```python
from build123d import *

# Parameters (mm, degrees)
SKETCH_1_W          = 12
SKETCH_1_H          = 10
EXTRUDE_1_DEPTH     = 9
FILLET_1_R          = 0.5
SKETCH_2_R          = 2
SKETCH_2_R_2        = 1.5
EXTRUDE_2_DEPTH     = 0.8
FILLET_2_R          = 0.05
SKETCH_7_R          = 2
CUT_EXTRUDE_4_DEPTH = 0.1


with BuildPart() as part:
    # 草图1 → 凸台-拉伸1 (new body)
    with BuildSketch(Plane.XY):
        Rectangle(SKETCH_1_W, SKETCH_1_H)
    extrude(amount=EXTRUDE_1_DEPTH)

    # 圆角1
    fillet_1_edges = [part.edges().sort_by_distance(p)[0] for p in [
        (6, -5, 4.5),
        (-6, -5, 4.5),
        (-6, 5, 4.5),
        (6, 5, 4.5),
    ]]
    fillet(fillet_1_edges, radius=FILLET_1_R)

    # 草图2 → 凸台-拉伸2 (add)
    with BuildSketch(Plane.XY.offset(9)):
        Circle(SKETCH_2_R)
        Circle(SKETCH_2_R_2, mode=Mode.SUBTRACT)
    extrude(amount=EXTRUDE_2_DEPTH)

    # 圆角2
    fillet_2_edges = [part.edges().sort_by_distance(p)[0] for p in [
        (-2, 0, 9.8),
    ]]
    fillet(fillet_2_edges, radius=FILLET_2_R)

    # 草图7 → 切除-拉伸4 (cut)
    with BuildSketch(Plane(origin=(0, 0, 0), x_dir=(-1, 0, 0), z_dir=(0, 0, -1))):
        Circle(SKETCH_7_R)
    extrude(amount=-CUT_EXTRUDE_4_DEPTH, mode=Mode.SUBTRACT)


solid = part.part
```
Input: part model. Units: mm. Frame: model coordinates. A direction names the side the tool comes from. Give positions to 0.01 mm unless a question says otherwise; leave off trailing zeros. Order: outer loops, then holes, each group sorted by start corner. A loop starts at its lowest first (then second) coordinate and runs counter-clockwise, first axis right, second up. Notation, with made-up numbers: M 24,89.5 L 69,89.5 A9 ccw 69,93.5 Z; hole C 60,-12.75 d3. An arc over 180 degrees is marked long. Return JSON: item names as keys, results as strings.
1) Section query C-C on x = 5.25. Output: boundary loops of the cut face in (y, z), and give its area (3 significant figures).
Taken from the geometry:
{"outline": "M -5,0 L 5,0 L 5,9 L -5,9 Z", "area": "90.0 mm2"}
2) Section query D-D on y = -4. Output: boundary loops of the cut face in (x, z).
Taken from the geometry:
{"outline": "M -6,0 L 6,0 L 6,9 L -6,9 Z"}
3) Section query B-B on x = 0. Output: boundary loops of the cut face in (y, z).
Taken from the geometry:
{"outline": "M -5,0 L -2,0 L -2,0.1 L 2,0.1 L 2,0 L 5,0 L 5,9 L 2,9 L 2,9.75 A0.05 ccw 1.95,9.8 L 1.5,9.8 L 1.5,9 L -1.5,9 L -1.5,9.8 L -1.95,9.8 A0.05 ccw -2,9.75 L -2,9 L -5,9 Z"}
4) Line query: L1, parallel to Y at x = 0, z = 0.05; L2, parallel to Y at x = 0, z = 9.2; L3, parallel to Z at x = -4, y = 0.5. Output: solid intervals per line, ascending. Write a range as [from, to].
Taken from the geometry:
{"L1": "y = [-5, -2], [2, 5]", "L2": "y = [-2, -1.5], [1.5, 2]", "L3": "z = [0, 9]"}
5) Access query for faces 1 (the face through (-0.1, 2.3, 0)), 2 (the face through (-0.1, 2.3, 9)). Directions: +Z, -Z, +X, -X, +Y, -Y. A direction counts if a zero-diameter tool reaches every point of the face in a straight line with its end or side. Return the directions, or none.
Taken from the geometry:
{"face 1": "-Z, +X, -X, +Y, -Y", "face 2": "+Z"}
6) Contact query for a flat-ended pin moving along its axis: pin 1 (1.5 mm diameter, centred on x = -0.5, y = 0.5, fed in from +Z). Output: stop coordinate, or through.
Taken from the geometry:
{"pin 1": "stops at z = 9"}
7) Mould query, pull axis Y, two halves, no side actions, for faces 3 (the face through (0, 0, 0.1)), 4 (the face through (-6, 0, 4)), 5 (the face through (-0.434, -1.952, 9.37)). Classes: released by +Y, released by -Y, zero draft, split by the parting line, or undercut.
Taken from the geometry:
{"face 3": "undercut", "face 4": "zero draft", "face 5": "split by the parting line"}
8) Section query A-A on y = 0. Output: boundary loops of the cut face in (x, z), and give its area (3 significant figures).
Taken from the geometry:
{"outline": "M -6,0 L -2,0 L -2,0.1 L 2,0.1 L 2,0 L 6,0 L 6,9 L 2,9 L 2,9.75 A0.05 ccw 1.95,9.8 L 1.5,9.8 L 1.5,9 L -1.5,9 L -1.5,9.8 L -1.95,9.8 A0.05 ccw -2,9.75 L -2,9 L -6,9 Z", "area": "108 mm2"}
